```python
from build123d import *

# Parameters (mm, degrees)
SKETCH1_W                                            = 280
SKETCH1_H                                            = 140
EXTRUDE1_DEPTH                                       = 20
M6_TAPPED_HOLE1_D                                    = 5
M6_TAPPED_HOLE2_D                                    = 5
M6_TAPPED_HOLE3_D                                    = 5
M6_TAPPED_HOLE3_DEPTH                                = 25
M6_TAPPED_HOLE3_TIP                                  = 1.502151548
CBORE_FOR_M6_HEX_SOCKET_THIN_HEAD_CAP_SC_D           = 6.6
CBORE_FOR_M6_HEX_SOCKET_THIN_HEAD_CAP_SC_CBORE_D     = 11
CBORE_FOR_M6_HEX_SOCKET_THIN_HEAD_CAP_SC_CBORE_DEPTH = 4.6
M6_TAPPED_HOLE4_D                                    = 5
M6_TAPPED_HOLE4_DEPTH                                = 25
M6_TAPPED_HOLE4_TIP                                  = 1.502151548


with BuildPart() as part:
    # Sketch1 → Extrude1 (new body)
    with BuildSketch(Plane(origin=(0, 0, 0), x_dir=(1, 0, 0), z_dir=(0, 1, 0))):
        Rectangle(SKETCH1_W, SKETCH1_H)
    extrude(amount=EXTRUDE1_DEPTH)

    # M6 Tapped Hole1 (through all)
    with Locations(Plane(origin=(0, 0, 0), x_dir=(-1, 0, 0), z_dir=(0, -1, 0))):
        with Locations((-110, 60), (-55, 60), (-110, 0), (-55, 0), (-110, -60), (-55, -60), (55, 60), (110, 60), (110, 0), (55, 0), (110, -60), (55, -60)):
            Hole(M6_TAPPED_HOLE1_D / 2)

    # M6 Tapped Hole2 (through all)
    with Locations(Plane(origin=(0, 20, 0), x_dir=(1, 0, 0), z_dir=(0, 1, 0))):
        with Locations((-91.5, 23), (-78.5, 23), (-91.5, -23), (-78.5, -23), (130, 23), (130, -23)):
            Hole(M6_TAPPED_HOLE2_D / 2)

    # M6 Tapped Hole3
    with Locations(Plane(origin=(140, 0, 0), x_dir=(0, 0, -1), z_dir=(1, 0, 0))):
        with Locations((-58, 10), (0, 10), (58, 10)):
            Hole(M6_TAPPED_HOLE3_D / 2, depth=M6_TAPPED_HOLE3_DEPTH)
            with Locations((0, 0, -(M6_TAPPED_HOLE3_DEPTH + M6_TAPPED_HOLE3_TIP / 2))):  # 118° drill point
                Cone(0, M6_TAPPED_HOLE3_D / 2, M6_TAPPED_HOLE3_TIP, mode=Mode.SUBTRACT)

    # CBORE for M6 Hex Socket Thin Head Cap Screw1 (through all)
    with Locations(Plane(origin=(0, 0, 0), x_dir=(-1, 0, 0), z_dir=(0, -1, 0))):
        with Locations((-125, 52.5), (-70, 52.5), (0, 52.5), (0, -52.5), (-70, -52.5), (-125, -52.5), (125, -52.5), (70, -52.5), (70, 52.5), (125, 52.5)):
            CounterBoreHole(CBORE_FOR_M6_HEX_SOCKET_THIN_HEAD_CAP_SC_D / 2, CBORE_FOR_M6_HEX_SOCKET_THIN_HEAD_CAP_SC_CBORE_D / 2, CBORE_FOR_M6_HEX_SOCKET_THIN_HEAD_CAP_SC_CBORE_DEPTH)

    # M6 Tapped Hole4
    with Locations(Plane.ZY.offset(140)):
        with Locations((58, 10), (0, 10), (-58, 10)):
            Hole(M6_TAPPED_HOLE4_D / 2, depth=M6_TAPPED_HOLE4_DEPTH)
            with Locations((0, 0, -(M6_TAPPED_HOLE4_DEPTH + M6_TAPPED_HOLE4_TIP / 2))):  # 118° drill point
                Cone(0, M6_TAPPED_HOLE4_D / 2, M6_TAPPED_HOLE4_TIP, mode=Mode.SUBTRACT)


solid = part.part
```
Design review of the part built by this model. Coordinates are the model's own, in mm. A direction names the side the tool comes from. Round coordinates to 2 decimals unless told otherwise and drop trailing zeros. Write each loop counter-clockwise with the first axis right and the second up, starting at its lowest first coordinate (ties: lowest second). Pieces come first, ordered by that corner, then holes.
Item 1: The part is to be moulded in two halves that separate along Z. For faces 1 (the flat face through (-2, 10, 70)), 2 (the flat face through (140, 5, 1)), 3 (the cylindrical face through (0.716, 2.268, 47.047)), say which applies: +Z half, -Z half, draft (parallel to the pull), parting line (faces both ways), or undercut.
Item 2: For probe 1 along Z at (x, y) = (55, 13); probe 2 along X at (y, z) = (2.05, -52.5); probe 3 along X at (y, z) = (9.25, -52.5), list the stretches that pass through material, from the lowest coordinate up.
Item 3: For faces 4 (the cylindrical face through (127.615, 9.86, -23.751)), 5 (the cylindrical face through (-127.3, 10.1, 60.5)), 6 (the flat face through (-74, 4.6, 52)), list the 3-axis set-ups (+Z, -Z, +X, -X, +Y, -Y) from which the entire face can be reached by the end or side of a thin tool; tool diameter is ignored.
Item 4: We need section A-A on x = -70. Write out the cut boundary in (y, z).
Item 5: We need section B-B on z = -52.5. State how many separate pieces and enclosed holes the cut face has, and give its area (3 significant figures).
Item 6: Clearance check with flat-ended pins moving along their axes: pin 1 Ø3.5 at (x, z) = (-0.5, 50.5) entering from -Y; pin 2 Ø3 at (y, z) = (10, 58) entering from -X; pin 3 Ø4.5 at (y, z) = (10, 58) entering from -X. State where each tip first meets the part, or that it passes through.
Returned:
1. face 1: +Z half
1. face 2: draft
1. face 3: undercut
2. probe 1: z = -70 to -62.5, -57.5 to -2.5, 2.5 to 57.5, 62.5 to 70
2. probe 2: x = -140 to -130.5, -119.5 to -75.5, -64.5 to -5.5, 5.5 to 64.5, 75.5 to 119.5, 130.5 to 140
2. probe 3: x = -140 to -128.3, -121.7 to -73.3, -66.7 to -3.3, 3.3 to 66.7, 73.3 to 121.7, 128.3 to 140
3. face 4: +Y, -Y
3. face 5: -X
3. face 6: -Y
4. outline: (0, -70) - (20, -70) - (20, -55.8) - (4.6, -55.8) - (4.6, -58) - (0, -58) - close; (0, -47) - (4.6, -47) - (4.6, -49.2) - (20, -49.2) - (20, 49.2) - (4.6, 49.2) - (4.6, 47) - (0, 47) - close; (0, 58) - (4.6, 58) - (4.6, 55.8) - (20, 55.8) - (20, 70) - (0, 70) - close
5. separate pieces: 6
5. enclosed holes: 0
5. area: 4,840 mm2
6. pin 1: stops at y = 4.6
6. pin 2: stops at x = -114.4
6. pin 3: stops at x = -114.85
